from build123d import *

# Parameters (mm, degrees)
F0_W     = 508
F0_H     = 609.6
F1_DEPTH = 19.05
F2_W     = 127
F2_H     = 609.6
F3_DEPTH = 19.05
F4_W     = 88.9
F4_H     = 609.6
F5_DEPTH = 19.05
F6_W     = 88.9
F6_H     = 609.6
F6_W_2   = 22.225
F6_W_3   = 111.125
F6_H_2   = 611.105501
F7_DEPTH = 19.05
F8_W     = 508
F8_H     = 609.6
F8_R     = 228.6
F9_DEPTH = 19.05
F10_D    = 12.7


with BuildPart() as f1:
    # F0 (on Front) → F1 (new body)
    with BuildSketch(Plane.XZ):
        Rectangle(F0_W, F0_H)
    extrude(amount=F1_DEPTH)

    # F2 (on face) → F3 (join)
    with BuildSketch(Plane(origin=(0, 0, 0), x_dir=(-1, 0, 0), z_dir=(0, 1, 0))):
        with Locations((177.8, 0)):
            Rectangle(F2_W, F2_H)
        with Locations((-177.8, 0)):
            Rectangle(F2_W, F2_H)
    extrude(amount=F3_DEPTH)

    # F4 (on face) → F5 (join)
    with BuildSketch(Plane(origin=(0, 19.05, 0), x_dir=(-1, 0, 0), z_dir=(0, 1, 0))):
        with Locations((196.85, 0)):
            Rectangle(F4_W, F4_H)
        with Locations((-196.85, 0.023927)):
            Rectangle(F4_W, F4_H)
    extrude(amount=F5_DEPTH)

    # F6 (on face) → F7 (join)
    with BuildSketch(Plane(origin=(0, 38.1, 0), x_dir=(-1, 0, 0), z_dir=(0, 1, 0))):
        with Locations((196.85, 0)):
            Rectangle(F6_W, F6_H)
        with Locations((141.2875, 0)):
            Rectangle(F6_W_2, F6_H)
        with Locations((-185.7375, -0.065833)):
            Rectangle(F6_W_3, F6_H_2)
    extrude(amount=F7_DEPTH)

    # F8 (on face) → F9 (join)
    with BuildSketch(Plane.XZ.offset(19.05)):
        Rectangle(F8_W, F8_H)
        Circle(F8_R, mode=Mode.SUBTRACT)
    extrude(amount=F9_DEPTH)

    # F10 (through all)
    with Locations(Plane.XZ.offset(19.05)):
        with Locations((0, 0)):
            Hole(F10_D / 2)


solid = f1.part
Work out the finished part from the listing and answer in its coordinate system (mm). A direction names the side the tool comes from. Give positions to 0.01 mm unless a question says otherwise; leave off trailing zeros. Loops run counter-clockwise (first coordinate to the right, second up) from the corner with the lowest first, then second, coordinate; pieces in that order, holes last. Notation, with made-up numbers: (47, 4) -> (87, 4) arc R16 cw to (87, 16) -> close; hole circle Ø4 at (11.5, 22.5). An arc over 180 degrees is marked (long way). Use a Markdown table: item, result. Add a question column.
1) The part is cut by section A-A, the plane y = 28.5. Determine the outline of the cut face in (x, z).
2) The part is cut by section D-D, the plane z = -39. Determine the outline of the cut face in (x, y) (3 decimals), plus the area to 3 significant figures.
3) Each of these flat-tipped pins is pushed along its axis until it touches: P1, Ø5, axis at y = 27, z = 218.5, coming from the +X side; P2, Ø15, axis at y = 8.5, z = 57, coming from the -X side; P3, Ø4, axis at x = -76.5, y = -9, coming from the +Z side; P4, Ø10, axis at x = -246, z = 13.5, coming from the +Y side. Where does it stop, or does it pass through?
4) Consider line 1 along Z through (x, y) = (0, -29); line 2 along X through (y, z) = (35, 114); line 3 along X through (y, z) = (9, 116). Determine where each line is inside the solid, lowest interval first.
5) For a pull along Z with two mould halves and no side action, classify faces 1 (the cylindrical face through (-228.38, -28.44, 10.05)), 2 (the flat face through (130.175, 47, -4)), 3 (the flat face through (197, 28, -304.776)) as +Z half, -Z half, draft (parallel to the pull), parting line (faces both ways), or undercut.
6) Which of the six approach directions +Z, -Z, +X, -X, +Y, -Y give full straight-line access (tool end or side, diameter ignored) to faces 4 (the flat face through (114.3, 9, -4)), 5 (the flat face through (-133, 19.05, 4)), 6 (the flat face through (248, 0, 4))?
7) The part is cut by section C-C, the plane x = -19. Determine the outline of the cut face in (y, z), plus the area to 3 significant figures.
Reported:
| question | item | result |
|---|---|---|
| 1 | outline | (-241.3, -304.8) -> (-152.4, -304.8) -> (-152.4, 304.8) -> (-241.3, 304.8) -> close; (152.4, -304.78) -> (241.3, -304.78) -> (241.3, 304.82) -> (152.4, 304.82) -> close |
| 2 | outline | (-254, -38.1) -> (-225.249, -38.1) -> (-225.249, -19.05) -> (225.249, -19.05) -> (225.249, -38.1) -> (254, -38.1) -> (254, 0) -> (241.3, 0) -> (241.3, 57.15) -> (130.175, 57.15) -> (130.175, 38.1) -> (152.4, 38.1) -> (152.4, 19.05) -> (114.3, 19.05) -> (114.3, 0) -> (-114.3, 0) -> (-114.3, 19.05) -> (-152.4, 19.05) -> (-152.4, 38.1) -> (-130.175, 38.1) -> (-130.175, 57.15) -> (-241.3, 57.15) -> (-241.3, 0) -> (-254, 0) -> close |
| 2 | area | 23,200 mm^2 |
| 3 | P1 | stops at x = 241.3 |
| 3 | P2 | stops at x = -241.3 |
| 3 | P3 | stops at z = 304.8 |
| 3 | P4 | stops at y = 57.15 |
| 4 | line 1 | z = -304.8 to -228.6, 228.6 to 304.8 |
| 4 | line 2 | x = -241.3 to -152.4, 152.4 to 241.3 |
| 4 | line 3 | x = -241.3 to -114.3, 114.3 to 241.3 |
| 5 | face 1 | undercut |
| 5 | face 2 | draft |
| 5 | face 3 | -Z half |
| 6 | face 4 | +Z, -Z, +Y |
| 6 | face 5 | +Z, -Z |
| 6 | face 6 | +Z, -Z, +X, +Y |
| 7 | outline | (-38.1, -304.8) -> (0, -304.8) -> (0, 304.8) -> (-38.1, 304.8) -> (-38.1, 227.81) -> (-19.05, 227.81) -> (-19.05, -227.81) -> (-38.1, -227.81) -> close |
| 7 | area | 14,500 mm^2 |
